Check sheet for the modelled part. Datum: model origin and axes. Units: mm. Coordinates: 2 decimals unless noted, no trailing zeros. Loops run counter-clockwise (first coordinate to the right, second up) from the corner with the lowest first, then second, coordinate; pieces in that order, holes last. Notation, with made-up numbers: (-30.5, -31.75) - (19.5, -31.75) arc R24 cw to (19.5, 6.25) - close; hole circle Ø9 at (73, -25). An arc over 180 degrees is marked (long way). Write each question's results on one line, items separated by ' | '. Start each with the question number.
1. Cross-section at B-B (y = -45.5). Record the cut outline in (x, z).
2. Cross-section at D-D (x = -42). Record the cut outline in (y, z), and give its area (3 significant figures).
3. Cross-section at C-C (z = 4.5). Record the cut outline in (x, y), and give its area (3 significant figures).
4. Cross-section at A-A (z = 41.5). Record the cut outline in (x, y), and give its area (3 significant figures).
5. Gauge pin test, flat ends, axial feed: P1, Ø5.5, axis at x = 26.5, z = 36, coming from the -Y side; P2, Ø3, axis at x = 2, z = 35.5, coming from the -Y side; P3, Ø14.5, axis at x = -23, z = 42.5, coming from the +Y side. Record the tip position at first contact, or that the pin passes through.
6. Draft check along X on faces 1 (the face through (-22, -53.34, 39)), 2 (the face through (29.213, -45.613, 42.029)), 3 (the face through (-18.866, -45.613, 45.984)), 4 (the face through (21.145, -45.613, 46.223)). Enter one of: released by +X, released by -X, zero draft, split by the parting line, or undercut.
7. Thickness scan on line 1 (Y direction, x = -24, z = -6.5); line 2 (X direction, y = 1.5, z = 22); line 3 (Z direction, x = -16, y = 48.5). Record the ranges inside material, lowest first. Write a range as [from, to].
```python
from build123d import *

# Parameters (mm, degrees)
F4_DEPTH = 15.24


with BuildPart() as f1:
    # F0 (on Front) → F1 (revolve)
    with BuildSketch(Plane.XZ):
        with BuildLine():
            Line((0, 56.691967), (0, -56.691967))
            ThreePointArc((0, -56.691967), (56.691967, 0), (0, 56.691967))
        make_face()
    revolve(axis=Axis((0, 0, 0.728689), (0, 0, -1)))

    # F3 (on offset) → F4 (join)
    with BuildSketch(Plane.XZ.offset(38.1)):
        Polygon((-22.443607, 59.023771), (-30.896394, 25.504097), (-13.407868, 26.087049), align=None)
        Polygon((24.483934, 59.023771), (15.739674, 25.504097), (33.811152, 25.504097), align=None)
    extrude(amount=F4_DEPTH)


solid = f1.part
```
Established:
1) outline: (-30.9, 25.5) - (-21.86, 25.81) arc R33.82 ccw (long way) to (22.21, 25.5) - (33.81, 25.5) - (24.48, 59.02) - (16.75, 29.38) arc R33.82 ccw to (-14.62, 30.5) - (-22.44, 59.02) - close
2) outline: circle Ø76.16 at (0, 0) | area: 4,560 mm^2
3) outline: circle Ø113.03 at (0, 0) | area: 10,000 mm^2
4) outline: circle Ø77.25 at (0, 0); (-26.86, -53.34) - (-17.64, -53.34) - (-17.64, -38.1) - (-26.86, -38.1) - close; (19.91, -53.34) - (29.36, -53.34) - (29.36, -38.1) - (19.91, -38.1) - close | area: 4,970 mm^2
5) P1: y = -53.34 | P2: y = -45.32 | P3: y = 39.08
6) face 1: zero draft | face 2: released by +X | face 3: undercut | face 4: undercut
7) line 1: [-50.95, 50.95] | line 2: [-52.23, 52.23] | line 3: [-24.61, 24.61]
